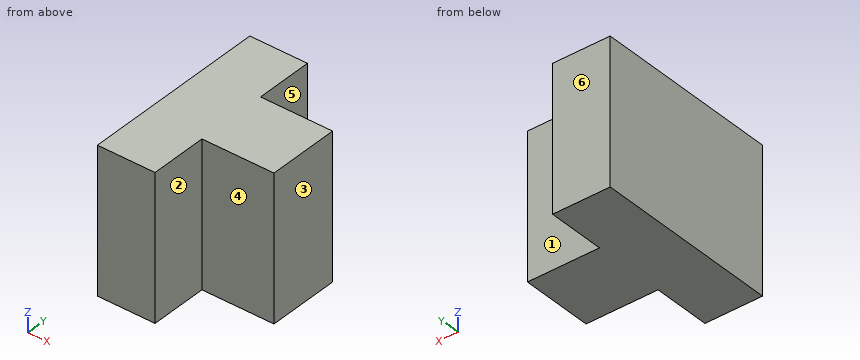
```python
from build123d import *

# Parameters (mm, degrees)
BOX028_W               = 1
BOX028_H               = 5
BOX028_DEPTH           = 10
BOX027_W               = 13
BOX027_H               = 15
BOX027_DEPTH           = 10
BOX026_W               = 4
BOX026_H               = 4
BOX026_DEPTH           = 17
BOX025_W               = 4
BOX025_H               = 4
BOX025_DEPTH           = 17
BOX024_W               = 8
BOX024_H               = 13
BOX024_DEPTH           = 13
CUT025_PLACEMENT_ANGLE = 180


with BuildPart() as cubo028:
    # Box028 → Box028 (new body)
    with BuildSketch(Plane(origin=(49, 4, 0), x_dir=(1, 0, 0), z_dir=(0, 0, 1))):
        with Locations((0.5, 2.5)):
            Rectangle(BOX028_W, BOX028_H)
    extrude(amount=BOX028_DEPTH)


with BuildPart() as cubo027:
    # Box027 → Box027 (new body)
    with BuildSketch(Plane(origin=(38, -1, 10), x_dir=(1, 0, 0), z_dir=(0, 0, 1))):
        with Locations((6.5, 7.5)):
            Rectangle(BOX027_W, BOX027_H)
    extrude(amount=BOX027_DEPTH)


with BuildPart() as cubo026:
    # Box026 → Box026 (new body)
    with BuildSketch(Plane(origin=(0, 9, 0), x_dir=(1, 0, 0), z_dir=(0, 0, 1))):
        with Locations((2, 2)):
            Rectangle(BOX026_W, BOX026_H)
    extrude(amount=BOX026_DEPTH)


with BuildPart() as cubo025:
    # Box025 → Box025 (new body)
    with BuildSketch(Plane.XY):
        with Locations((2, 2)):
            Rectangle(BOX025_W, BOX025_H)
    extrude(amount=BOX025_DEPTH)


with BuildPart() as obj1:
    # Box024 → Box024 (new body)
    with BuildSketch(Plane.XY):
        with Locations((4, 6.5)):
            Rectangle(BOX024_W, BOX024_H)
    extrude(amount=BOX024_DEPTH)

    # Cut024: cut Cubo025
    add(cubo025.part, mode=Mode.SUBTRACT)

    # Cut025: cut Cubo026
    add(cubo026.part, mode=Mode.SUBTRACT)


with BuildPart() as obj1_1:
    # Cut025 placement: moved
    add(obj1.part.moved(Location((50, 13, 0))).rotate(Axis((50, 13, 0), (0, 0, 1)), CUT025_PLACEMENT_ANGLE))

    # Cut026: cut Cubo027
    add(cubo027.part, mode=Mode.SUBTRACT)


with BuildPart() as obj1_2:
    # Cut026 placement: moved
    add(obj1_1.part.moved(Location((-1, 0, 0))))

    # Fusion014: union Cubo028
    add(cubo028.part)


solid = obj1_2.part
```
The model under review builds one solid part; all positions refer to its coordinate system, in mm. Face numbers are marked on the shaded views. A direction names the side the tool comes from. Coordinates: 2 decimals unless noted, no trailing zeros. Write each loop counter-clockwise with the first axis right and the second up, starting at its lowest first coordinate (ties: lowest second). Pieces come first, ordered by that corner, then holes. Notation, with made-up numbers: (64.5, 27.5) - (75.5, 27.5) arc R13 ccw to (75.5, 47.5) - close; hole circle Ø2 at (24, -8). An arc over 180 degrees is marked (long way). Answer in a Markdown table with one row per item. Add a question column.
Q1. For the marked faces 1, 2 and 3, list the 3-axis set-ups (+Z, -Z, +X, -X, +Y, -Y) from which the entire face can be reached by the end or side of a thin tool; tool diameter is ignored.
Q2. Draft analysis for pull direction Y (two halves, no side actions). For the marked faces 4, 5 and 6, state which applies: +Y half, -Y half, draft (parallel to the pull), parting line (faces both ways), or undercut.
Q3. To check wall thickness, follow line 1 along X through (y, z) = (9.75, 4.25); line 2 along Y through (x, z) = (47.25, 6.25). State the ranges of each line that lie inside material, in increasing order. Write a range as from..to.
Q4. Consider section B-B on x = 47.5. Give the boundary of the cut face in (y, z), then the cut area to 3 significant figures.
Q5. Consider section A-A on z = 6. Give the boundary of the cut face in (x, y), then the cut area to 3 significant figures.
Q6. Consider section C-C on y = 10.5. Give the boundary of the cut face in (x, z), then the cut area to 3 significant figures.
Q7. Clearance check with flat-ended pins moving along their axes: pin 1 (3 mm diameter, centred on y = 10, z = 4, fed in from +X); pin 2 (4.5 mm diameter, centred on y = 1.5, z = 5, fed in from +X). State where each tip first meets the part, or that it passes through.
Answers below:
| question | item | result |
|---|---|---|
| 1 | face 1 | +Z, -Z, +X, +Y |
| 1 | face 2 | +Z, -Z, +X, -Y |
| 1 | face 3 | +Z, -Z, +X, +Y, -Y |
| 2 | face 4 | -Y half |
| 2 | face 5 | draft |
| 2 | face 6 | +Y half |
| 3 | line 1 | 41..45 |
| 3 | line 2 | 4..9 |
| 4 | outline | (4, 0) - (9, 0) - (9, 10) - (4, 10) - close |
| 4 | area | 50.0 mm² |
| 5 | outline | (41, 0) - (45, 0) - (45, 4) - (50, 4) - (50, 9) - (45, 9) - (45, 13) - (41, 13) - close |
| 5 | area | 77.0 mm² |
| 6 | outline | (41, 0) - (45, 0) - (45, 10) - (41, 10) - close |
| 6 | area | 40.0 mm² |
| 7 | pin 1 | x = 50 |
| 7 | pin 2 | x = 45 |
